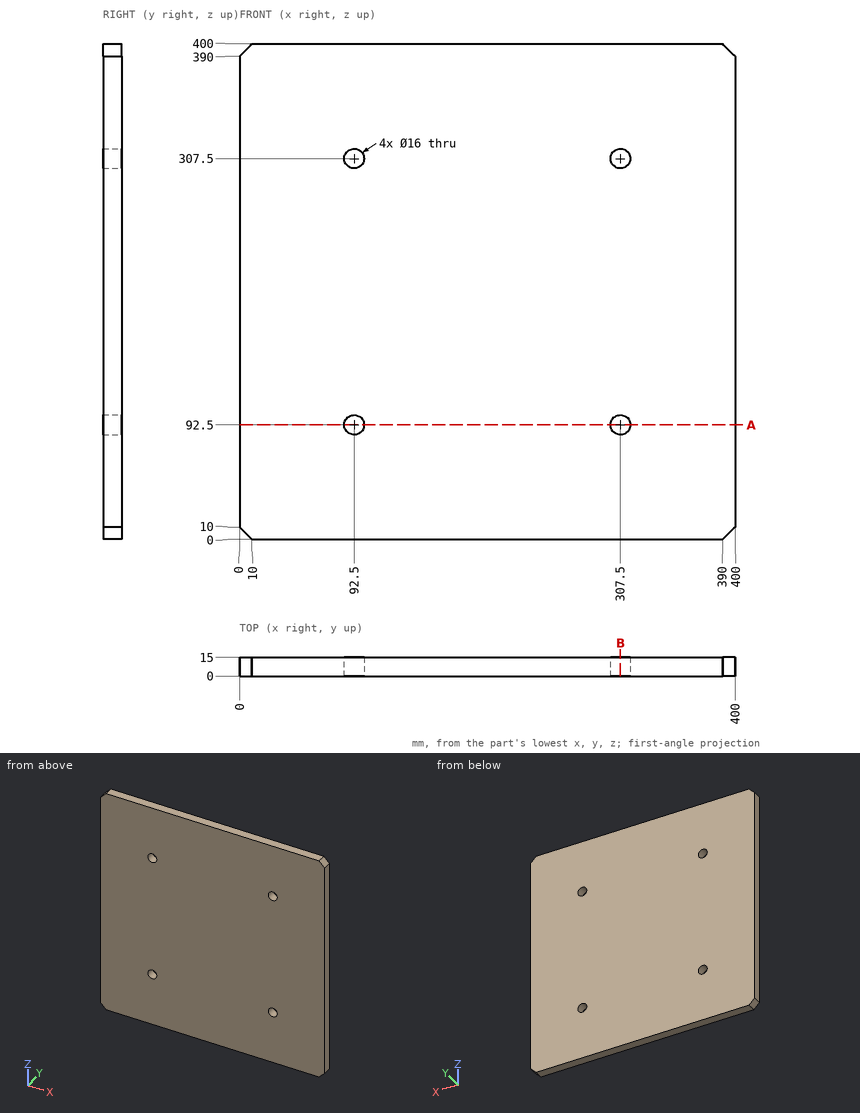
Geometry check sheet. Reference: drawing and pictorial views, mm from the part's lowest x, y, z. Give positions to 0.01 mm unless a question says otherwise; leave off trailing zeros. Order: outer loops, then holes, each group sorted by start corner. A loop starts at its lowest first (then second) coordinate and runs counter-clockwise, first axis right, second up. Notation, with made-up numbers: M 18,38.25 L 26,38.25 A18 cw 26,63.25 Z; hole C 5,-38 d4. An arc over 180 degrees is marked long. Answer in a Markdown table with one row per item. Add a question column.
Q1. Sectioned sample at B-B, the plane x = 307.5. Record the boundary of the cut face in (y, z).
Q2. Thickness scan on L1, parallel to Z at x = 307.5, y = 4.25; L2, parallel to X at y = 1, z = 311. Record the ranges inside material, lowest first.
Q3. Sectioned sample at A-A, the plane z = 92.5. Record the boundary of the cut face in (x, y), and give its area (3 significant figures).
Verdict:
| question | item | result |
|---|---|---|
| 1 | outline | M 0,0 L 15,0 L 15,84.5 L 0,84.5 Z; M 0,100.5 L 15,100.5 L 15,299.5 L 0,299.5 Z; M 0,315.5 L 15,315.5 L 15,400 L 0,400 Z |
| 2 | L1 | 0 to 84.5, 100.5 to 299.5, 315.5 to 400 |
| 2 | L2 | 0 to 85.31, 99.69 to 300.31, 314.69 to 400 |
| 3 | outline | M 0,0 L 84.5,0 L 84.5,15 L 0,15 Z; M 100.5,0 L 299.5,0 L 299.5,15 L 100.5,15 Z; M 315.5,0 L 400,0 L 400,15 L 315.5,15 Z |
| 3 | area | 5,520 mm² |
